from build123d import *

# Parameters (mm, degrees)
F1_DEPTH = 300
F2_R     = 50


with BuildPart() as f1:
    # F0 (on Top) → F1 (new body)
    with BuildSketch(Plane.XY):
        Polygon((-260.881037, 629.978729), (-260.881037, -1120.021271), (39.118963, -1120.021271), (39.118963, 629.978729), (489.118963, 1079.978729), (249.118963, 1079.978729), (39.118963, 869.978729), (39.118963, 1079.978729), (-260.881037, 1079.978729), (-260.881037, 869.978729), (-470.881037, 1079.978729), (-710.881037, 1079.978729), align=None)
    extrude(amount=F1_DEPTH)

    # F2
    f2_edges = [f1.edges().sort_by_distance(p)[0] for p in [
        (-260.881037, -245.021271, 300),
        (39.118963, -245.021271, 300),
        (39.118963, -245.021271, 0),
        (-260.881037, -245.021271, 0),
        (39.118963, 974.978729, 0),
        (-260.881037, 974.978729, 0),
        (39.118963, 974.978729, 300),
        (-260.881037, 974.978729, 300),
        (-365.881037, 974.978729, 300),
        (-485.881037, 854.978729, 300),
        (264.118963, 854.978729, 300),
        (264.118963, 854.978729, 0),
        (144.118963, 974.978729, 0),
        (-365.881037, 974.978729, 0),
        (-485.881037, 854.978729, 0),
        (144.118963, 974.978729, 300),
    ]]
    fillet(f2_edges, radius=F2_R)


solid = f1.part
Design review of the part built by this model. Coordinates are the model's own, in mm. A direction names the side the tool comes from. Round coordinates to 2 decimals unless told otherwise and drop trailing zeros. Write each loop counter-clockwise with the first axis right and the second up, starting at its lowest first coordinate (ties: lowest second). Pieces come first, ordered by that corner, then holes. Notation, with made-up numbers: (30.25, 59) - (54.25, 59) arc R8 cw to (54.25, 74) - close; hole circle Ø6 at (23.5, -17). An arc over 180 degrees is marked (long way). Use a Markdown table: item, result. Add a question column.
1. Wall thickness on probe 1 along X at (y, z) = (-861.5, 229.5); probe 2 along Z at (x, y) = (-415, 989); probe 3 along Y at (x, z) = (439.5, 220.5): over which ranges is each line inside the solid? List them lowest first.
2. Clearance check with flat-ended pins moving along their axes: pin 1 (3 mm diameter, centred on y = 21, z = 261, fed in from -X); pin 2 (3 mm diameter, centred on y = -453, z = 178.5, fed in from -X); pin 3 (4 mm diameter, centred on y = 859.5, z = 172, fed in from +X). State where each tip first meets the part, or that it passes through.
3. Mouldability with a two-part tool opening along X and no side actions: class faces 4 (the face through (-113, -1120.021, 148)), 5 (the face through (39.119, -257, 149)), 6 (the face through (-260.881, -233, 149)), 7 (the face through (126.886, 937.582, 284.964)) as +X half, -X half, draft (parallel to the pull), parting line (faces both ways), or undercut.
4. For faces 1 (the face through (24.861, -222.271, 284.964)), 2 (the face through (-246.623, -247.061, 15.036)), 3 (the face through (-246.623, 949.054, 15.036)), list the 3-axis set-ups (+Z, -Z, +X, -X, +Y, -Y) from which the entire face can be reached by the end or side of a thin tool; tool diameter is ignored.
5. We need section B-B (y = -136.5). State the section outline as (x, z) points, then the cut area to 3 significant figures.
6. We need section A-A (z = 175). State the section outline as (x, y) points, then the cut area to 3 significant figures.
Output:
| question | item | result |
|---|---|---|
| 1 | probe 1 | x = -260.88 to 39.12 |
| 1 | probe 2 | z = 6.8 to 293.2 |
| 1 | probe 3 | y = 1030.36 to 1079.98 |
| 2 | pin 1 | stops at x = -259.97 |
| 2 | pin 2 | stops at x = -260.88 |
| 2 | pin 3 | stops at x = 270.64 |
| 3 | face 4 | draft |
| 3 | face 5 | +X half |
| 3 | face 6 | -X half |
| 3 | face 7 | undercut |
| 4 | face 1 | +Z, +X, -Y |
| 4 | face 2 | -Z, -X, -Y |
| 4 | face 3 | -Z, +Y |
| 5 | outline | (-260.88, 50) arc R50 ccw to (-210.88, 0) - (-10.88, 0) arc R50 ccw to (39.12, 50) - (39.12, 250) arc R50 ccw to (-10.88, 300) - (-210.88, 300) arc R50 ccw to (-260.88, 250) - close |
| 5 | area | 87,900 mm2 |
| 6 | outline | (-710.88, 1079.98) - (-260.88, 629.98) - (-260.88, -1120.02) - (39.12, -1120.02) - (39.12, 629.98) - (489.12, 1079.98) - (249.12, 1079.98) - (39.12, 869.98) - (39.12, 1079.98) - (-260.88, 1079.98) - (-260.88, 869.98) - (-470.88, 1079.98) - close |
| 6 | area | 818,000 mm2 |
